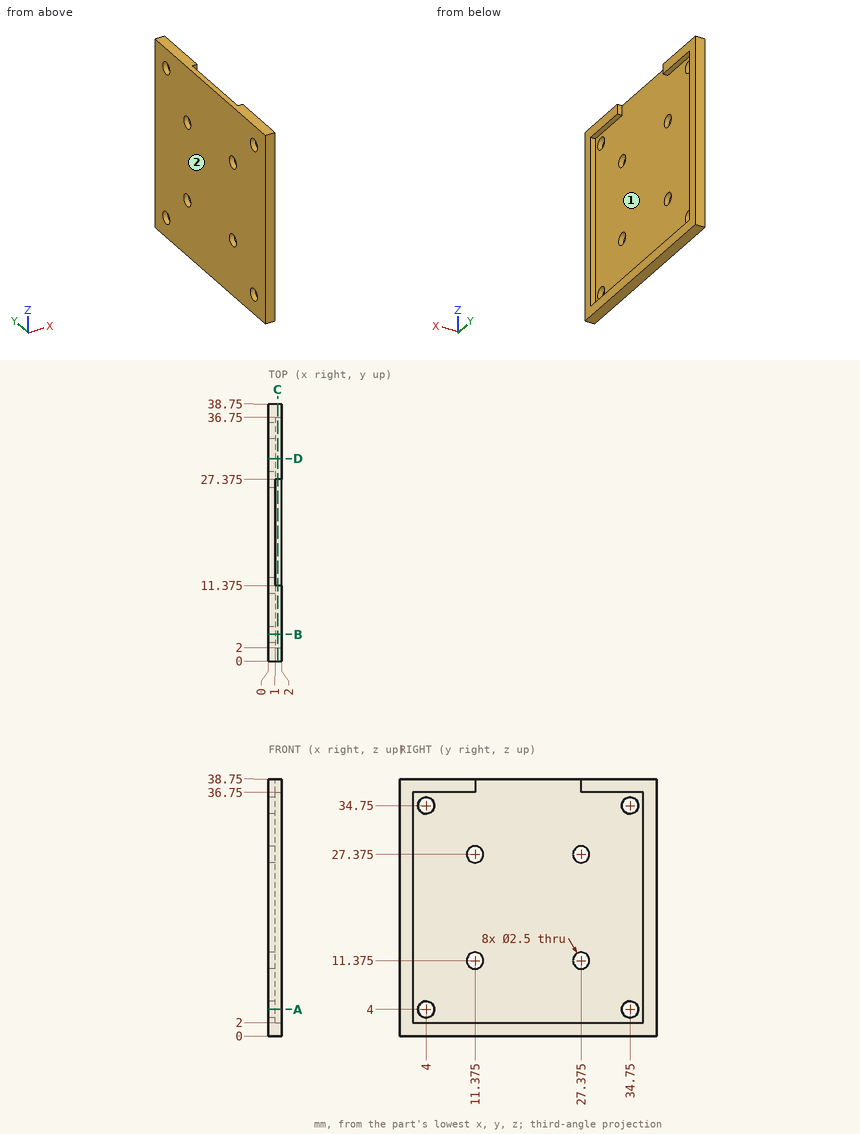
Design review of the part shown in the three views and the two pictorial views. Dimensions are in mm from the part's minimum x, y and z. Coordinates: 2 decimals unless noted, no trailing zeros. Loops run counter-clockwise (first coordinate to the right, second up) from the corner with the lowest first, then second, coordinate; pieces in that order, holes last. Notation, with made-up numbers: M 23.5,-14 L 47.5,-14 A27 cw 47.5,25 Z; hole C -21.5,24.5 d11. An arc over 180 degrees is marked long. Put each result on its own line as item: value. Start each with the question number.
Q1. Add section D-D (y = 30.5). Write out the cut boundary in (x, z).
Q2. Clearance check with flat-ended pins moving along their axes: pin 1 (3 mm diameter, centred on y = 27.375, z = 11.375, fed in from +X); pin 2 (2 mm diameter, centred on y = 34.75, z = 34.75, fed in from +X). State where each tip first meets the part, or that it passes through.
Q3. Add section C-C (x = 1.4). Write out the cut boundary in (y, z) (3 decimals), and give its area (3 significant figures).
Q4. The part is to be moulded in two halves that separate along Y. For the marked faces 1 and 2, say which applies: +Y half, -Y half, draft (parallel to the pull), parting line (faces both ways), or undercut.
Q5. Add section A-A (z = 4). Write out the cut boundary in (x, y), and give its area (4 significant figures).
Q6. Wall thickness on line 1 (Z direction, x = 0.5, y = 4); line 2 (Y direction, x = 1.05, z = 34): over which ranges is each line inside the solid? List them lowest first.
Answers:
1. outline: M 0,0 L 2,0 L 2,2 L 1,2 L 1,36.75 L 2,36.75 L 2,38.75 L 0,38.75 Z
2. pin 1: stops at x = 1
2. pin 2: passes through
3. outline: M 0,0 L 38.75,0 L 38.75,38.75 L 27.375,38.75 L 27.375,36.75 L 36.75,36.75 L 36.75,2 L 2,2 L 2,36.75 L 11.375,36.75 L 11.375,38.75 L 0,38.75 Z
3. area: 262 mm^2
4. face 1: undercut
4. face 2: draft
5. outline: M 0,0 L 2,0 L 2,2 L 1,2 L 1,2.75 L 0,2.75 Z; M 0,5.25 L 1,5.25 L 1,33.5 L 0,33.5 Z; M 0,36 L 1,36 L 1,36.75 L 2,36.75 L 2,38.75 L 0,38.75 Z
5. area: 37.75 mm^2
6. line 1: z = 0 to 2.75, 5.25 to 33.5, 36 to 38.75
6. line 2: y = 0 to 2, 36.75 to 38.75
